Check sheet for the modelled part. Datum: model origin and axes. Units: mm. A direction names the side the tool comes from. Give positions to 0.01 mm unless a question says otherwise; leave off trailing zeros. Write each loop counter-clockwise with the first axis right and the second up, starting at its lowest first coordinate (ties: lowest second). Pieces come first, ordered by that corner, then holes. Notation, with made-up numbers: M 0,38.25 L 37,38.25 A19 cw 37,57.25 Z; hole C -24,72.25 d4. An arc over 180 degrees is marked long. Write item = value, one per line. Start each with the question number.
1) Sectioned sample at C-C, the plane y = 17.5. Record the cut outline in (x, z), then the cut area to 3 significant figures.
2) Set-up check for faces 5 (the face through (0, 0, 50)), 6 (the face through (-4.336, 19.524, 34.79)): record each of +Z, -Z, +X, -X, +Y, -Y from which the full face is reachable in a straight line by a thin tool's end or side.
3) Sectioned sample at A-A, the plane x = 0. Record the cut outline in (y, z), then the cut area to 3 significant figures.
4) Sectioned sample at D-D, the plane z = 32.5. Record the cut outline in (x, y), then the cut area to 3 significant figures.
5) Gauge pin test, flat ends, axial feed: pin 1 (6 mm diameter, centred on x = -11.5, z = 42, fed in from -Y); pin 2 (1 mm diameter, centred on x = 28, y = 40, fed in from +Z); pin 3 (12 mm diameter, centred on x = -7.5, z = 35, fed in from +Y). Record the tip position at first contact, or that the pin passes through.
6) Scan lines: L1, parallel to Z at x = 6, y = -15; L2, parallel to Z at x = -59, y = 8; L3, parallel to Y at x = 43, z = 3.5. Record each from-to range of solid material in increasing order.
7) Draft check along Z on faces 1 (the face through (4.2, 0.3, 20)), 2 (the face through (-1, 1, 0)), 3 (the face through (-0.867, 3.905, 14.93)), 4 (the face through (-16.04, 72.24, 4.93)). Enter one of: pulls with the +Z half, pulls with the -Z half, needs draft (parallel to the pull), parting line crosses it, or undercut.
Autodesk Inventor part; units mm, degrees
ref_plane "YZ Plane" through (0, 0, 0) normal (1, 0, 0) x (0, 1, 0)
ref_plane "XZ Plane" through (0, 0, 0) normal (0, 1, 0) x (-1, 0, 0)
ref_plane "XY Plane" through (0, 0, 0) normal (0, 0, 1) x (1, 0, 0)
sketch "Sketch1" plane through (0, 0, 0) normal (0, 0, 1) x (1, 0, 0)
  circle A0 centre (0, 0) radius 74
extrude "Extrusion1" add sketch "Sketch1" along normal blind 10
sketch "Sketch2" plane through (0, 0, 10) normal (0, 0, 1) x (1, 0, 0)
  circle A0 centre (0, 0) radius 4
  dimension "d3" = 8
extrude "Extrusion2" add sketch "Sketch2" along normal blind 10
sketch "Sketch3" plane through (0, 0, 20) normal (0, 0, 1) x (1, 0, 0)
  circle A0 centre (0, 0) radius 4
  circle A1 centre (0, 0) radius 20
  dimension "d6" = 40
extrude "Extrusion3" add sketch "Sketch3" along normal blind 30 contours A0 | A1
properties part number "Project_Rough_disc"
Data:
q1.outline = M -71.9,0 L 71.9,0 L 71.9,10 L -71.9,10 Z; M -9.68,20 L 9.68,20 L 9.68,50 L -9.68,50 Z
q1.area = 2,020 mm2
q2.face_5 = +Z, +X, -X, +Y, -Y
q2.face_6 = +Z
q3.outline = M -74,0 L 74,0 L 74,10 L 4,10 L 4,20 L 20,20 L 20,50 L -20,50 L -20,20 L -4,20 L -4,10 L -74,10 Z
q3.area = 2,760 mm2
q4.outline = C 0,0 d40
q4.area = 1,260 mm2
q5.pin_1 = -18.1
q5.pin_2 = 10
q5.pin_3 = 19.94
q6.L1 = 0 to 10, 20 to 50
q6.L2 = 0 to 10
q6.L3 = -60.22 to 60.22
q7.face_1 = undercut
q7.face_2 = pulls with the -Z half
q7.face_3 = undercut
q7.face_4 = needs draft
